Model file for the job. Use its own axes, mm. A direction names the side the tool comes from. Round coordinates to 2 decimals unless told otherwise and drop trailing zeros. Loops run counter-clockwise (first coordinate to the right, second up) from the corner with the lowest first, then second, coordinate; pieces in that order, holes last.
from build123d import *

# Parameters (mm, degrees)
SKETCH_1_W             = 46.2
SKETCH_1_H             = 34.2
EXTRUDE_1_DEPTH        = 22
SHELL_1_T              = -2
CUT_EXTRUDE_3_REACH    = 55.952
SKETCH_4_W             = 30.2
SKETCH_4_H             = 2
SKETCH_5_W             = 31.8
SKETCH_5_H             = 1
CUT_EXTRUDE_4_DEPTH    = 45
CUT_EXTRUDE_6_REACH    = 38.194
SKETCH_8_W             = 14
SKETCH_8_H             = 2
CUT_EXTRUDE_7_REACH    = 48.768
SKETCH_9_W             = 14
SKETCH_9_H             = 2
FILLET_3_R             = 1
FILLET_4_R             = 1
FILLET_3_OF_MIRROR_1_R = 1
FILLET_4_OF_MIRROR_1_R = 1
CUT_EXTRUDE_8_REACH    = 55.952
SKETCH_10_W            = 10
SKETCH_10_H            = 4.5
FILLET_6_R             = 0.4
CUT_EXTRUDE_9_REACH    = 55.952
SKETCH_11_W            = 11
SKETCH_11_H            = 5
FILLET_7_R             = 0.4
CUT_EXTRUDE_10_REACH   = 55.952
SKETCH_12_R            = 1.25


# Some blends are built 0.0001 mm under size
with BuildPart() as part:
    # 草图1 → 凸台-拉伸1 (new body)
    with BuildSketch(Plane(origin=(0, 0, 0), x_dir=(1, 0, 0), z_dir=(0, 1, 0))):
        Rectangle(SKETCH_1_W, SKETCH_1_H)
    extrude(amount=EXTRUDE_1_DEPTH)

    # 抽壳1
    shell_1_openings = [part.faces().sort_by_distance(p)[0] for p in [
        (0, 22, 0),
    ]]
    offset(amount=SHELL_1_T, openings=shell_1_openings, kind=Kind.INTERSECTION)

    # 草图4 → 切除-拉伸3 (cut, up to next)
    with BuildSketch(Plane(origin=(23.1, 0, 0), x_dir=(0, 0, -1), z_dir=(1, 0, 0)), mode=Mode.PRIVATE) as cut_extrude_3_sk1:
        with Locations((0, 21)):
            Rectangle(SKETCH_4_W, SKETCH_4_H)
    cut_extrude_3_tool1 = extrude(cut_extrude_3_sk1.sketch, amount=-CUT_EXTRUDE_3_REACH, mode=Mode.PRIVATE) & part.part
    add(cut_extrude_3_tool1.solids().sort_by_distance((23.1, 21, 0))[0], mode=Mode.SUBTRACT)

    # 草图5 → 切除-拉伸4 (cut)
    with BuildSketch(Plane(origin=(23.1, 0, 0), x_dir=(0, 0, -1), z_dir=(1, 0, 0))):
        with Locations((0, 20.5)):
            Rectangle(SKETCH_5_W, SKETCH_5_H)
    extrude(amount=-CUT_EXTRUDE_4_DEPTH, mode=Mode.SUBTRACT)

    # 草图8 → 切除-拉伸6 (cut, up to next)
    with BuildSketch(Plane.XZ, mode=Mode.PRIVATE) as cut_extrude_6_sk1:
        with Locations((0, -14.1)):
            Rectangle(SKETCH_8_W, SKETCH_8_H)
    cut_extrude_6_tool1 = extrude(cut_extrude_6_sk1.sketch, amount=-CUT_EXTRUDE_6_REACH, mode=Mode.PRIVATE) & part.part
    cut_extrude_6 = cut_extrude_6_tool1.solids().sort_by_distance((0, 0, -14.1))[0]
    add(cut_extrude_6, mode=Mode.SUBTRACT)

    # 草图9 → 切除-拉伸7 (cut, up to next)
    with BuildSketch(Plane(origin=(0, 0, -17.1), x_dir=(-1, 0, 0), z_dir=(0, 0, -1)), mode=Mode.PRIVATE) as cut_extrude_7_sk1:
        with Locations((0, 3)):
            Rectangle(SKETCH_9_W, SKETCH_9_H)
    cut_extrude_7_tool1 = extrude(cut_extrude_7_sk1.sketch, amount=-CUT_EXTRUDE_7_REACH, mode=Mode.PRIVATE) & part.part
    cut_extrude_7 = cut_extrude_7_tool1.solids().sort_by_distance((0, 3, -17.1))[0]
    add(cut_extrude_7, mode=Mode.SUBTRACT)

    # 圆角3
    # the kernel refuses this fillet: 1 mm, written as the material it adds along each edge
    with BuildSketch(Plane(origin=(-7, 4, -17.1), x_dir=(0, -1, 0), z_dir=(0, 0, 1)), Plane(origin=(-7, 2, -17.1), x_dir=(1, 0, 0), z_dir=(0, 0, 1)), Plane(origin=(7, 2, -17.1), x_dir=(0, 1, 0), z_dir=(0, 0, 1))) as fillet_3_piece_1:
        with BuildLine():
            CenterArc((FILLET_3_R, FILLET_3_R), FILLET_3_R, 180, 90)
            Line((0, FILLET_3_R), (0, 0))
            Line((0, 0), (FILLET_3_R, 0))
        make_face()
    extrude(amount=2)
    with BuildSketch(Plane(origin=(7, 4, -17.1), x_dir=(0, -1, 0), z_dir=(0, 0, 1))) as fillet_3_piece_2:
        with BuildLine():
            CenterArc((FILLET_3_R, -FILLET_3_R), FILLET_3_R, 90, 90)
            Line((0, -FILLET_3_R), (0, 0))
            Line((0, 0), (FILLET_3_R, 0))
        make_face()
    extrude(amount=2)

    # 圆角4
    fillet_4_edges = [part.edges().sort_by_distance(p)[0] for p in [
        (-7, 1, -15.1),
        (-7, 1, -13.1),
        (7, 1, -15.1),
        (7, 1, -13.1),
    ]]
    fillet(fillet_4_edges, radius=FILLET_4_R - 0.0001)  # a hair under: the kernel refuses the full size

    # 镜向1: 切除-拉伸6, 切除-拉伸7 across plane
    add(cut_extrude_6.mirror(Plane.XY), mode=Mode.SUBTRACT)
    add(cut_extrude_7.mirror(Plane.XY), mode=Mode.SUBTRACT)

    # 圆角3 of 镜向1
    # the kernel refuses this fillet: 1 mm, written as the material it adds along each edge
    with BuildSketch(Plane(origin=(-7, 4, 17.1), x_dir=(1, 0, 0), z_dir=(0, 0, -1)), Plane(origin=(-7, 2, 17.1), x_dir=(0, 1, 0), z_dir=(0, 0, -1)), Plane(origin=(7, 2, 17.1), x_dir=(-1, 0, 0), z_dir=(0, 0, -1))) as fillet_3_of_mirror_1_piece_1:
        with BuildLine():
            CenterArc((FILLET_3_OF_MIRROR_1_R, FILLET_3_OF_MIRROR_1_R), FILLET_3_OF_MIRROR_1_R, 180, 90)
            Line((0, FILLET_3_OF_MIRROR_1_R), (0, 0))
            Line((0, 0), (FILLET_3_OF_MIRROR_1_R, 0))
        make_face()
    extrude(amount=2)
    with BuildSketch(Plane(origin=(7, 4, 17.1), x_dir=(-1, 0, 0), z_dir=(0, 0, -1))) as fillet_3_of_mirror_1_piece_2:
        with BuildLine():
            CenterArc((FILLET_3_OF_MIRROR_1_R, -FILLET_3_OF_MIRROR_1_R), FILLET_3_OF_MIRROR_1_R, 90, 90)
            Line((0, -FILLET_3_OF_MIRROR_1_R), (0, 0))
            Line((0, 0), (FILLET_3_OF_MIRROR_1_R, 0))
        make_face()
    extrude(amount=2)

    # 圆角4 of 镜向1
    fillet_4_of_mirror_1_edges = [part.edges().sort_by_distance(p)[0] for p in [
        (-7, 1, 15.1),
        (-7, 1, 13.1),
        (7, 1, 15.1),
        (7, 1, 13.1),
    ]]
    fillet(fillet_4_of_mirror_1_edges, radius=FILLET_4_OF_MIRROR_1_R - 0.0001)  # a hair under: the kernel refuses the full size

    # 草图10 → 切除-拉伸8 (cut, up to next)
    with BuildSketch(Plane.ZY.offset(23.1), mode=Mode.PRIVATE) as cut_extrude_8_sk1:
        with Locations((-10.1, 12.75)):
            Rectangle(SKETCH_10_W, SKETCH_10_H)
    cut_extrude_8_tool1 = extrude(cut_extrude_8_sk1.sketch, amount=-CUT_EXTRUDE_8_REACH, mode=Mode.PRIVATE) & part.part
    add(cut_extrude_8_tool1.solids().sort_by_distance((-23.1, 12.75, -10.1))[0], mode=Mode.SUBTRACT)

    # 圆角6
    fillet_6_edges = [part.edges().sort_by_distance(p)[0] for p in [
        (-22.1, 10.5, -5.1),
        (-22.1, 15, -5.1),
        (-22.1, 15, -15.1),
        (-22.1, 10.5, -15.1),
    ]]
    fillet(fillet_6_edges, radius=FILLET_6_R)

    # 草图11 → 切除-拉伸9 (cut, up to next)
    with BuildSketch(Plane.ZY.offset(23.1), mode=Mode.PRIVATE) as cut_extrude_9_sk1:
        with Locations((5.6, 14.5)):
            Rectangle(SKETCH_11_W, SKETCH_11_H)
    cut_extrude_9_tool1 = extrude(cut_extrude_9_sk1.sketch, amount=-CUT_EXTRUDE_9_REACH, mode=Mode.PRIVATE) & part.part
    add(cut_extrude_9_tool1.solids().sort_by_distance((-23.1, 14.5, 5.6))[0], mode=Mode.SUBTRACT)

    # 圆角7
    fillet_7_edges = [part.edges().sort_by_distance(p)[0] for p in [
        (-22.1, 17, 0.1),
        (-22.1, 12, 0.1),
        (-22.1, 12, 11.1),
        (-22.1, 17, 11.1),
    ]]
    fillet(fillet_7_edges, radius=FILLET_7_R)

    # 草图12 → 切除-拉伸10 (cut, up to next)
    with BuildSketch(Plane(origin=(23.1, 0, 0), x_dir=(0, 0, -1), z_dir=(1, 0, 0)), mode=Mode.PRIVATE) as cut_extrude_10_sk1:
        with Locations((-2.9, 16)):
            Circle(SKETCH_12_R)
    cut_extrude_10_tool1 = extrude(cut_extrude_10_sk1.sketch, amount=-CUT_EXTRUDE_10_REACH, mode=Mode.PRIVATE) & part.part
    # 草图12 → 切除-拉伸10 (cut, up to next)
    with BuildSketch(Plane(origin=(23.1, 0, 0), x_dir=(0, 0, -1), z_dir=(1, 0, 0)), mode=Mode.PRIVATE) as cut_extrude_10_sk2:
        with Locations((1.1, 16)):
            Circle(SKETCH_12_R)
    cut_extrude_10_tool2 = extrude(cut_extrude_10_sk2.sketch, amount=-CUT_EXTRUDE_10_REACH, mode=Mode.PRIVATE) & part.part
    add(cut_extrude_10_tool1.solids().sort_by_distance((23.1, 16, 2.9))[0], mode=Mode.SUBTRACT)
    add(cut_extrude_10_tool2.solids().sort_by_distance((23.1, 16, -1.1))[0], mode=Mode.SUBTRACT)


solid = part.part
Q1. Slice it at B-B on y = 3. Give the cut face in (x, z), plus the area to 3 significant figures.
Q2. Slice it at D-D on y = 16. Give the cut face in (x, z).
Q3. Probe line 1 (X direction, y = 7.5, z = -4.5); line 2 (Z direction, x = -9.5, y = 5.5); line 3 (Y direction, x = 22, z = -1). List the from-to ranges inside material, lowest first.
Q4. Tool access for faces 5 (the face through (-7, 3, 16)), 6 (the face through (6.699, 1.014, 13.385)), 7 (the face through (-22, 17, 6)), 8 (the face through (-21.1, 9, 0)), 9 (the face through (0.7, 21, 15.4)): list every direction of +Z, -Z, +X, -X, +Y, -Y with a clear straight run to the whole face (end or side of a thin tool).
Q5. Slice it at A-A on z = 2.9. Give the cut face in (x, y).
Q6. Flat gauge pin, fed straight in: P1, Ø0.5, axis at y = 20.5, z = 2, coming from the +X side. Where does the tip first touch, or does it go through?
Q7. Pull direction X, two halves, no side cores. Call faces 1 (the face through (0, 1, -13.1)), 2 (the face through (-23.1, 11, 0)), 3 (the face through (0.7, 21.5, 15.1)), 4 (the face through (-6.699, 1.014, -14.815)): pulls with the +X half, pulls with the -X half, needs draft (parallel to the pull), parting line crosses it, or undercut.
Q8. Slice it at C-C on x = -5.5. Give the cut face in (y, z), plus the area to 3 significant figures.
Reply:
1. outline: (-23.1, -17.1) - (-7, -17.1) - (-7, -15.1) - (-21.1, -15.1) - (-21.1, 15.1) - (-7, 15.1) - (-7, 17.1) - (-23.1, 17.1) - close; (7, -17.1) - (23.1, -17.1) - (23.1, 17.1) - (7, 17.1) - (7, 15.1) - (21.1, 15.1) - (21.1, -15.1) - (7, -15.1) - close
1. area: 250 mm2
2. outline: (-23.1, -17.1) - (23.1, -17.1) - (23.1, -2.35) - (21.1, -2.35) - (21.1, -15.1) - (-21.1, -15.1) - (-21.1, 0.1) - (-23.1, 0.1) - close; (-23.1, 11.1) - (-21.1, 11.1) - (-21.1, 15.1) - (21.1, 15.1) - (21.1, 4.15) - (23.1, 4.15) - (23.1, 17.1) - (-23.1, 17.1) - close; (21.1, 0.15) - (23.1, 0.15) - (23.1, 1.65) - (21.1, 1.65) - close
3. line 1: x = -23.1 to -21.1, 21.1 to 23.1
3. line 2: z = -17.1 to -15.1, 15.1 to 17.1
3. line 3: y = 0 to 14.75, 17.25 to 20
4. face 5: +Z, -Z
4. face 6: +Y, -Y
4. face 7: -X
4. face 8: +Y
4. face 9: +X
5. outline: (-23.1, 0) - (23.1, 0) - (23.1, 14.75) - (21.1, 14.75) - (21.1, 2) - (-21.1, 2) - (-21.1, 12) - (-23.1, 12) - close; (-23.1, 17) - (-21.1, 17) - (-21.1, 20) - (-21.9, 20) - (-21.9, 21) - (-21.1, 21) - (-21.1, 22) - (-23.1, 22) - close; (21.1, 17.25) - (23.1, 17.25) - (23.1, 20) - (21.1, 20) - close
6. P1: stops at x = -21.9
7. face 1: undercut
7. face 2: pulls with the -X half
7. face 3: needs draft
7. face 4: undercut
8. outline: (0, -17.1) - (2, -17.1) - (2, -15.1) - (0, -15.1) - close; (0, -13.1) - (2, -13.1) - (2, 13.1) - (0, 13.1) - close; (0, 15.1) - (2, 15.1) - (2, 17.1) - (0, 17.1) - close; (4, -17.1) - (22, -17.1) - (22, -15.1) - (21, -15.1) - (21, -15.9) - (20, -15.9) - (20, -15.1) - (4, -15.1) - close; (4, 15.1) - (20, 15.1) - (20, 15.9) - (21, 15.9) - (21, 15.1) - (22, 15.1) - (22, 17.1) - (4, 17.1) - close
8. area: 131 mm2
